from build123d import *

# Parameters (mm, degrees)
BOSS_EXTRUDE1_DEPTH      = 30
BOSS_EXTRUDE1_DEPTH_BACK = 30
SKETCH1_W                = 76.52
SKETCH1_H                = 85.68
SKETCH1_W_2              = 60.52
SKETCH1_H_2              = 69.68
SKETCH2_R                = 2
CUT_EXTRUDE1_DEPTH       = 30
SKETCH3_R                = 3
CUT_EXTRUDE2_DEPTH       = 30
CHAMFER1_SIZE            = 12


with BuildPart() as part:
    # Sketch1 → Boss-Extrude1 (new, two sides: drawn at the far end of the back side and taken through both)
    with BuildSketch(Plane(origin=(0, 0, 0), x_dir=(0, 0, -1), z_dir=(1, 0, 0)).offset(-BOSS_EXTRUDE1_DEPTH_BACK)):
        with Locations((38.26, 42.84)):
            Rectangle(SKETCH1_W, SKETCH1_H)
        with Locations((38.26, 42.84)):
            Rectangle(SKETCH1_W_2, SKETCH1_H_2, mode=Mode.SUBTRACT)
    extrude(amount=BOSS_EXTRUDE1_DEPTH + BOSS_EXTRUDE1_DEPTH_BACK)

    # Sketch2 → Cut-Extrude1 (cut)
    with BuildSketch(Plane(origin=(0, 0, -76.52), x_dir=(-1, 0, 0), z_dir=(0, 0, -1))):
        with Locations((0, 71.68)):
            Circle(SKETCH2_R)
        with Locations((18, 49.18)):
            Circle(SKETCH2_R)
        with Locations((-18, 49.18)):
            Circle(SKETCH2_R)
        with Locations((0, 26.68)):
            Circle(SKETCH2_R)
    extrude(amount=-CUT_EXTRUDE1_DEPTH, mode=Mode.SUBTRACT)

    # Sketch3 → Cut-Extrude2 (cut)
    with BuildSketch(Plane.XY):
        with Locations((17.67766953, 22.32233047)):
            Circle(SKETCH3_R)
        with Locations((-17.67766953, 22.32233047)):
            Circle(SKETCH3_R)
        with Locations((-17.67766953, 57.67766953)):
            Circle(SKETCH3_R)
        with Locations((17.67766953, 57.67766953)):
            Circle(SKETCH3_R)
    extrude(amount=-CUT_EXTRUDE2_DEPTH, mode=Mode.SUBTRACT)

    # Chamfer1
    chamfer1_edges = [part.edges().sort_by_distance(p)[0] for p in [
        (0, 77.68, -8),
        (0, 8, -68.52),
    ]]
    chamfer(chamfer1_edges, length=CHAMFER1_SIZE)


solid = part.part
Geometry check sheet. Reference: the model listing, model coordinates, mm. A direction names the side the tool comes from. Give positions to 0.01 mm unless a question says otherwise; leave off trailing zeros. Loops run counter-clockwise (first coordinate to the right, second up) from the corner with the lowest first, then second, coordinate; pieces in that order, holes last. Notation, with made-up numbers: M 8.5,16 L 41.5,16 A19 cw 41.5,44 Z; hole C 80.25,19 d9. An arc over 180 degrees is marked long. Answer as a JSON object with one key per item and string values. Group by question number.
Item 1: Sectioned sample at B-B on y = 67.5. Record the boundary of the cut face in (x, z), plus the area to 3 significant figures.
Item 2: Mould release check, pull along Z, two halves, no side actions. Record for faces 6 (the flat face through (0, 77.68, -44)), 7 (the flat face through (-0.42, 14.08, -62.6)), 8 (the flat face through (0, 42, 0)), 9 (the cylindrical face through (15.297, 20.497, -3.944)): pulls with the +Z half, pulls with the -Z half, needs draft (parallel to the pull), parting line crosses it, or undercut.
Item 3: Sectioned sample at C-C on z = -40. Record the boundary of the cut face in (x, y), plus the area to 3 significant figures.
Item 4: Access from +Z, -Z, +X, -X, +Y, -Y to the whole of each face (thin tool, end or side, straight path). Record for faces 1 (the cylindrical face through (-18.07, 60.65, -3.94)), 2 (the flat face through (0, 0, -38)), 3 (the flat face through (-0.42, 71.6, -13.92)), 4 (the flat face through (0, 42, -76.52)), 5 (the cylindrical face through (-17.74, 51.163, -72.576)).
Item 5: Gauge pin test, flat ends, axial feed: pin 1 (3 mm diameter, centred on x = 18, y = 49.18, fed in from -Z); pin 2 (5.5 mm diameter, centred on x = 17.68, y = 22.32, fed in from +Z). Record the tip position at first contact, or that the pin passes through.
Item 6: Sectioned sample at A-A on x = 0. Record the boundary of the cut face in (y, z).
Item 7: Material ranges on L1, parallel to Y at x = 26, z = -25.5; L2, parallel to Z at x = -9, y = 40; L3, parallel to Z at x = -24, y = 14.5, recorded low to high.
Item 8: Sectioned sample at D-D on x = -22. Record the boundary of the cut face in (y, z), plus the area to 3 significant figures.
Findings below:
{
 "1": {"outline": "M -30,-76.52 L 30,-76.52 L 30,-68.52 L -30,-68.52 Z; M -30,-9.82 L 30,-9.82 L 30,0 L -30,0 Z", "area": "1,070 mm2"},
 "2": {"face 6": "undercut", "face 7": "undercut", "face 8": "pulls with the +Z half", "face 9": "needs draft"},
 "3": {"outline": "M -30,0 L 30,0 L 30,8 L -30,8 Z; M -30,77.68 L 30,77.68 L 30,85.68 L -30,85.68 Z", "area": "960 mm2"},
 "4": {"face 1": "+Z", "face 2": "+Z, -Z, +X, -X, -Y", "face 3": "+X, -X", "face 4": "-Z, +X, -X, +Y, -Y", "face 5": "-Z"},
 "5": {"pin 1": "z = -8", "pin 2": "z = -68.09"},
 "6": {"outline": "M 0,-76.52 L 24.68,-76.52 L 24.68,-68.52 L 20,-68.52 L 8,-56.52 L 8,-8 L 65.68,-8 L 77.68,-20 L 77.68,-68.52 L 73.68,-68.52 L 73.68,-76.52 L 85.68,-76.52 L 85.68,0 L 0,0 Z; M 28.68,-76.52 L 69.68,-76.52 L 69.68,-68.52 L 28.68,-68.52 Z"},
 "7": {"L1": "0 to 8, 77.68 to 85.68", "L2": "-76.52 to -68.52, -8 to 0", "L3": "-76.52 to -63.02, -8 to 0"},
 "8": {"outline": "M 0,-76.52 L 85.68,-76.52 L 85.68,0 L 0,0 Z; hole M 8,-56.52 L 20,-68.52 L 77.68,-68.52 L 77.68,-20 L 65.68,-8 L 8,-8 Z", "area": "2,480 mm2"}
}
